Build history of the part. All positions in model axes, mm. Give positions to 0.01 mm unless a question says otherwise; leave off trailing zeros. Loops run counter-clockwise (first coordinate to the right, second up) from the corner with the lowest first, then second, coordinate; pieces in that order, holes last. Notation, with made-up numbers: M 50.5,38 L 89.5,38 A9 cw 89.5,51 Z; hole C 26,50.5 d7. An arc over 180 degrees is marked long. Answer as a JSON object with one key per item and string values. Group by question number.
1. Slice it at B-B (y = -50). List the corners of the cut face in (x, z), then the cut area to 3 significant figures.
2. Slice it at A-A (z = 2.25). Give the number of separate pieces and of enclosed holes in the cut face, then the cut area to 3 significant figures.
3. Drop a flat-ended pin along its axis: pin 1 Ø5 at (x, y) = (349.25, -247.65) entering from -Z. Give the stop position or say it passes through.
4. Drill centre lines: line 1 along X through (y, z) = (260.35, 3.75) (3 decimals); line 2 along Y through (x, z) = (349.25, 3.5) (3 decimals); line 3 along X through (y, z) = (196.85, 5). Where is each one in solid material? Low to high. Write a range as [from, to].
from build123d import *

# Parameters (mm, degrees)
SKETCH1_W                   = 736.6
SKETCH1_H                   = 596.9
BOSS_EXTRUDE1_DEPTH         = 6.35
SKETCH5_W                   = 31.75
SKETCH5_H                   = 76.2
BOSS_EXTRUDE2_DEPTH         = 6.35
SKETCH6_W                   = 6.35
SKETCH6_H                   = 444.5
CUT_EXTRUDE1_DEPTH          = 7.35
FILLET1_R                   = 6.35
F_0_257_DIAMETER_HOLE1_D    = 6.5278
F_1_4_0_25_DIAMETER_HOLE2_D = 6.35
CUT_EXTRUDE2_DEPTH          = 7.35


with BuildPart() as part:
    # Sketch1 → Boss-Extrude1 (new body)
    with BuildSketch(Plane.XY):
        Rectangle(SKETCH1_W, SKETCH1_H)
    extrude(amount=BOSS_EXTRUDE1_DEPTH)

    # Sketch5 → Boss-Extrude2 (add)
    with BuildSketch(Plane.XY.offset(6.35)):
        with Locations((-384.175, 260.35)):
            Rectangle(SKETCH5_W, SKETCH5_H)
        with Locations((-384.175, -260.35)):
            Rectangle(SKETCH5_W, SKETCH5_H)
    extrude(amount=-BOSS_EXTRUDE2_DEPTH)

    # Sketch6 → Cut-Extrude1 (cut, through all)
    with BuildSketch(Plane.XY.offset(6.35)):
        with Locations((-365.125, 0)):
            Rectangle(SKETCH6_W, SKETCH6_H)
    extrude(amount=-CUT_EXTRUDE1_DEPTH, mode=Mode.SUBTRACT)

    # Fillet1
    fillet1_edges = [part.edges().sort_by_distance(p)[0] for p in [
        (-361.95, -222.25, 3.175),
        (-361.95, 222.25, 3.175),
    ]]
    fillet(fillet1_edges, radius=FILLET1_R)

    # F (0.257) Diameter Hole1 (through all)
    with Locations(Plane.XY.offset(6.35)):
        with Locations((349.25, 247.65), (349.25, 196.85), (349.25, -196.85), (349.25, -247.65)):
            Hole(F_0_257_DIAMETER_HOLE1_D / 2)

    # 1/4 (0.25) Diameter Hole2 (through all)
    with Locations(Plane.XY.offset(6.35)):
        with Locations((-387.35, 260.35), (-361.95, 260.35), (-361.95, -241.3), (-387.35, -241.3)):
            Hole(F_1_4_0_25_DIAMETER_HOLE2_D / 2)

    # Sketch13 → Cut-Extrude2 (cut, through all)
    with BuildSketch(Plane.XY.offset(6.35)):
        with BuildLine():
            Line((368.3, 298.45), (342.9, 298.45))
            Line((342.9, 298.45), (342.9, 288.925))
            ThreePointArc((342.9, 288.925), (344.759871939, 284.434871939), (349.25, 282.575))
            Line((349.25, 282.575), (368.3, 282.575))
            Line((368.3, 282.575), (368.3, 298.45))
        make_face()
    extrude(amount=-CUT_EXTRUDE2_DEPTH, mode=Mode.SUBTRACT)


solid = part.part
Established:
{
 "1": {"outline": "M -361.95,0 L 368.3,0 L 368.3,6.35 L -361.95,6.35 Z", "area": "4,640 mm^2"},
 "2": {"separate pieces": "1", "enclosed holes": "8", "area": "441,000 mm^2"},
 "3": {"pin 1": "passes through"},
 "4": {"line 1": "x = [-400.05, -390.525], [-384.175, -365.125], [-358.775, 368.3]", "line 2": "y = [-298.45, -250.914], [-244.386, -200.114], [-193.586, 193.586], [200.114, 244.386], [250.914, 282.575]", "line 3": "x = [-361.95, 345.99], [352.51, 368.3]"}
}
